from build123d import *

# Parameters (mm, degrees)
BOSS_EXTRUDE1_DEPTH = 20
SKETCH2_R           = 1.5
CUT_EXTRUDE1_DEPTH  = 20
SKETCH3_R           = 1.75
CUT_EXTRUDE2_DEPTH  = 5
FILLET1_R           = 2
SKETCH4_R           = 2.5
SKETCH4_R_2         = 1.5
BOSS_EXTRUDE2_DEPTH = 1.5


with BuildPart() as part:
    # Sketch1 → Boss-Extrude1 (new body)
    with BuildSketch(Plane.XY):
        Polygon((0, 0), (0, 28), (4, 28), (4, 4), (19, 4), (19, 0), align=None)
    extrude(amount=BOSS_EXTRUDE1_DEPTH)

    # Sketch2 → Cut-Extrude1 (cut, through all)
    with BuildSketch(Plane.ZY):
        with Locations((17.5, 10)):
            Circle(SKETCH2_R)
        with Locations((2.5, 10)):
            Circle(SKETCH2_R)
    extrude(amount=-CUT_EXTRUDE1_DEPTH, mode=Mode.SUBTRACT)

    # Sketch3 → Cut-Extrude2 (cut, through all)
    with BuildSketch(Plane(origin=(0, 4, 0), x_dir=(1, 0, 0), z_dir=(0, 1, 0))):
        with Locations((14, -4)):
            Circle(SKETCH3_R)
        with Locations((14, -16)):
            Circle(SKETCH3_R)
    extrude(amount=-CUT_EXTRUDE2_DEPTH, mode=Mode.SUBTRACT)

    # Fillet1
    fillet1_edges = [part.edges().sort_by_distance(p)[0] for p in [
        (4, 4, 10),
        (2, 28, 20),
        (2, 28, 0),
        (19, 2, 0),
        (19, 2, 20),
    ]]
    fillet(fillet1_edges, radius=FILLET1_R)

    # Sketch4 → Boss-Extrude2 (add)
    with BuildSketch(Plane.ZY):
        with Locations((2.5, 10)):
            Circle(SKETCH4_R)
        with Locations((2.5, 10)):
            Circle(SKETCH4_R_2, mode=Mode.SUBTRACT)
        with Locations((17.5, 10)):
            Circle(SKETCH4_R)
        with Locations((17.5, 10)):
            Circle(SKETCH4_R_2, mode=Mode.SUBTRACT)
    extrude(amount=BOSS_EXTRUDE2_DEPTH)


solid = part.part
Work out the finished part from the listing and answer in its coordinate system (mm). A direction names the side the tool comes from. Give positions to 0.01 mm unless a question says otherwise; leave off trailing zeros. Loops run counter-clockwise (first coordinate to the right, second up) from the corner with the lowest first, then second, coordinate; pieces in that order, holes last. Notation, with made-up numbers: M 60.25,-6 L 93.25,-6 A13 cw 93.25,13 Z; hole C -26.75,59.25 d2. An arc over 180 degrees is marked long. Use CSV: the item, a comma, the result in double quotes.
1) Find section C-C on z = 12. Write down the section's boundary in (x, y), plus the area to 3 significant figures.
Answer:
outline,"M 0,0 L 19,0 L 19,4 L 6,4 A2 cw 4,6 L 4,28 L 0,28 Z"
area,"173 mm^2"
2) Given P1, Ø1.5, axis at y = 9, z = 11, coming from the -X side; P2, Ø3.5, axis at y = 10, z = 17.5, coming from the +X side; P3, Ø2.5, axis at y = 10, z = 17.5, coming from the +X side, each flat-ended and moving along its own axis, determine where each tip first touches the part or whether it passes through.
Answer:
P1,"x = 0"
P2,"x = 4"
P3,"through"
3) Find section B-B on y = 10.75. Write down the section's boundary in (x, z), plus the area to 3 significant figures.
Answer:
outline,"M -1.5,0.12 L 0,0.12 L 0,0 L 4,0 L 4,1.2 L -1.5,1.2 Z; M -1.5,3.8 L 4,3.8 L 4,16.2 L -1.5,16.2 L -1.5,15.12 L 0,15.12 L 0,4.88 L -1.5,4.88 Z; M -1.5,18.8 L 4,18.8 L 4,20 L 0,20 L 0,19.88 L -1.5,19.88 Z"
area,"65.7 mm^2"
4) Find section D-D on x = 14. Write down the section's boundary in (y, z), plus the area to 3 significant figures.
Answer:
outline,"M 0,0 L 4,0 L 4,2.25 L 0,2.25 Z; M 0,5.75 L 4,5.75 L 4,14.25 L 0,14.25 Z; M 0,17.75 L 4,17.75 L 4,20 L 0,20 Z"
area,"52.0 mm^2"
5) Find section A-A on x = 1.25. Write down the section's boundary in (y, z).
Answer:
outline,"M 0,0 L 26,0 A2 ccw 28,2 L 28,18 A2 ccw 26,20 L 0,20 Z; hole C 10,2.5 d3; hole C 10,17.5 d3"
6) Consider L1, parallel to Z at x = 14, y = 2.9; L2, parallel to Y at x = -0.7, z = 17.5; L3, parallel to Y at x = 12.25, z = 10.75. Determine where each line is inside the solid, lowest interval first.
Answer:
L1,"0 to 2.25, 5.75 to 14.25, 17.75 to 20"
L2,"7.5 to 8.5, 11.5 to 12.5"
L3,"0 to 4"
7) Which of the six approach directions +Z, -Z, +X, -X, +Y, -Y give full straight-line access (tool end or side, diameter ignored) to faces 1 (the flat face through (12, 4, 10)), 2 (the cylindrical face through (18.4, 1.97, 0.57)), 3 (the cylindrical face through (-0.74, 7.56, 1.96))?
Answer:
face 1,"+Z, -Z, +X, +Y"
face 2,"-Z, +X, +Y, -Y"
face 3,"-X"
8) Determine the mould class of faces 4 (the cylindrical face through (13.772, 2.028, 14.265)), 5 (the cylindrical face through (15.617, 2.028, 4.67)), 6 (the flat face through (-1.5, 9, 19)), 7 (the cylindrical face through (2.03, 27.4, 19.43)) for opening direction X: released by +X, released by -X, zero draft, split by the parting line, or undercut.
Answer:
face 4,"undercut"
face 5,"undercut"
face 6,"released by -X"
face 7,"zero draft"
